For this review, use the dimensioned drawing (mm, ordinates from the lowest corner) and the shaded views. Coordinates: 2 decimals unless noted, no trailing zeros. Order: outer loops, then holes, each group sorted by start corner. A loop starts at its lowest first (then second) coordinate and runs counter-clockwise, first axis right, second up. Notation, with made-up numbers: M 50.25,24.5 L 93.25,24.5 A12 cw 93.25,33.5 Z; hole C 31.5,24.5 d6. An arc over 180 degrees is marked long. Answer in a Markdown table with one row per item.
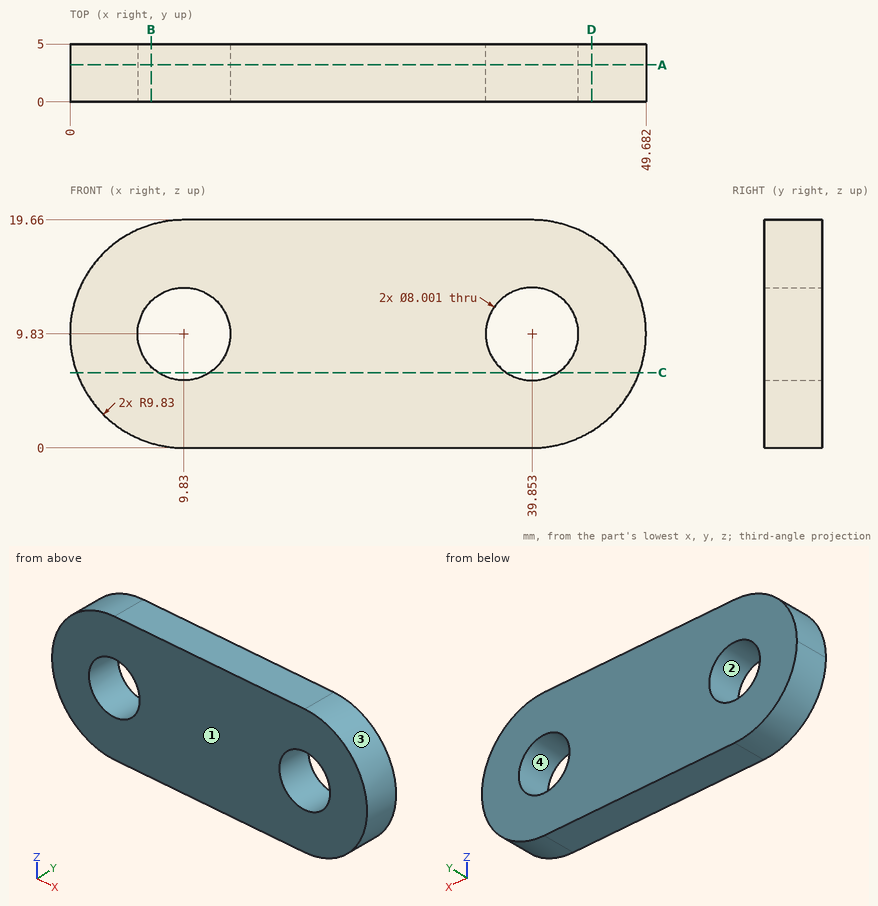
(1) The part is to be moulded in two halves that separate along X. For the marked faces 1, 2, 3 and 4, say which applies: +X half, -X half, draft (parallel to the pull), parting line (faces both ways), or undercut.
Report:
| item | result |
|---|---|
| face 1 | draft |
| face 2 | undercut |
| face 3 | +X half |
| face 4 | undercut |
(2) Insertion check: P1, Ø2, axis at y = 4.5, z = 2.5, coming from the +X side. The pin has a flat end and moves straight along its axis. Give the tip position at first contact, or say it passes through.
Report:
| item | result |
|---|---|
| P1 | x = 47.37 |
(3) Take a section at C-C (z = 6.5). Write out the cut boundary in (x, y) (1 decimal), then the cut area to 3 significant figures.
Report:
| item | result |
|---|---|
| outline | M 0.6,0 L 7.6,0 L 7.6,5 L 0.6,5 Z; M 12,0 L 37.6,0 L 37.6,5 L 12,5 Z; M 42.1,0 L 49.1,0 L 49.1,5 L 42.1,5 Z |
| area | 198 mm^2 |
(4) Take a section at D-D (x = 45). Write out the cut boundary in (y, z) (1 decimal).
Report:
| item | result |
|---|---|
| outline | M 0,1.5 L 5,1.5 L 5,18.2 L 0,18.2 Z |
(5) Take a section at B-B (x = 7). Write out the cut boundary in (y, z).
Report:
| item | result |
|---|---|
| outline | M 0,0.42 L 5,0.42 L 5,7 L 0,7 Z; M 0,12.66 L 5,12.66 L 5,19.24 L 0,19.24 Z |
(6) To check wall thickness, follow line 1 (X direction, y = 3.9, z = 7) (1 decimal); line 2 (X direction, y = 0.9, z = 13) (1 decimal); line 3 (Z direction, x = 43, y = 1.3) (1 decimal). State the ranges of each line that lie inside material, in increasing order. Write a range as [from, to].
Report:
| item | result |
|---|---|
| line 1 | [0.4, 7], [12.7, 37], [42.7, 49.3] |
| line 2 | [0.5, 7.4], [12.3, 37.4], [42.3, 49.2] |
| line 3 | [0.5, 7.4], [12.3, 19.1] |
(7) Take a section at A-A (y = 3.2). Write out the cut boundary in (x, z).
Report:
| item | result |
|---|---|
| outline | M 0,9.83 A9.83 ccw 9.83,0 L 39.85,0 A9.83 ccw 39.85,19.66 L 9.83,19.66 A9.83 ccw Z; hole C 9.83,9.83 d8; hole C 39.85,9.83 d8 |
